```python
from build123d import *

# Parameters (mm, degrees)
CROQUIS1_R              = 37.5
CROQUIS1_R_2            = 35
SALIENTE_EXTRUIR1_DEPTH = 15
CROQUIS2_R              = 40
SALIENTE_EXTRUIR2_DEPTH = 2
CORTAR_EXTRUIR1_DEPTH   = 10
CROQUIS5_W              = 2
CROQUIS5_H              = 4
SALIENTE_EXTRUIR3_START = -2
CROQUIS8_R              = 35
CROQUIS8_R_2            = 34
SALIENTE_EXTRUIR3_DEPTH = 7
REDONDEO1_R             = 0.5


with BuildPart() as part:
    # Croquis1 → Saliente-Extruir1 (new body)
    with BuildSketch(Plane(origin=(0, 17, 0), x_dir=(1, 0, 0), z_dir=(0, 1, 0))):
        with Locations(Location((13.541348433, 6.626768313, 0), (0, 0, 270))):
            Circle(CROQUIS1_R)
        with Locations(Location((13.541348433, 6.626768313, 0), (0, 0, 270))):
            Circle(CROQUIS1_R_2, mode=Mode.SUBTRACT)
    extrude(amount=SALIENTE_EXTRUIR1_DEPTH)

    # Croquis2 → Saliente-Extruir2 (add)
    with BuildSketch(Plane(origin=(0, 32, 0), x_dir=(1, 0, 0), z_dir=(0, 1, 0))):
        with Locations(Location((13.541348433, 6.626768313, 0), (0, 0, 270))):
            Circle(CROQUIS2_R)
    extrude(amount=SALIENTE_EXTRUIR2_DEPTH)

    # Croquis7 → Cortar-Extruir1 (cut)
    with BuildSketch(Plane.XZ.offset(-32)):
        with BuildLine():
            Line((13.541348433, -41.626768313), (13.541348433, -11.626768313))
            ThreePointArc((13.541348433, -11.626768313), (10.005814527, -10.162302219), (8.541348433, -6.626768313))
            Line((8.541348433, -6.626768313), (-21.458651567, -6.626768313))
            ThreePointArc((-21.458651567, -6.626768313), (-11.207388908, -31.375505654), (13.541348433, -41.626768313))
        make_face()
        with BuildLine():
            Line((48.541348433, -6.626768313), (18.541348433, -6.626768313))
            ThreePointArc((18.541348433, -6.626768313), (17.076882339, -3.091234407), (13.541348433, -1.626768313))
            Line((13.541348433, -1.626768313), (13.541348433, 28.373231687))
            ThreePointArc((13.541348433, 28.373231687), (38.290085775, 18.121969029), (48.541348433, -6.626768313))
        make_face()
    extrude(amount=-CORTAR_EXTRUIR1_DEPTH, mode=Mode.SUBTRACT)

    # Cortar-Barrer1: sweep along a path in Croquis6
    with BuildLine(Plane(origin=(0, 33, 0), x_dir=(1, 0, 0), z_dir=(0, 1, 0))) as cortar_barrer1_path:
        CenterArc((13.541348433, 6.626768313), 36.25, 0, 360)
    # Croquis5 → Cortar-Barrer1 (sweep, cut)
    with BuildSketch(Plane.XY.offset(-6.626768313)):
        with Locations((-22.208651567, 32.1)):
            Rectangle(CROQUIS5_W, CROQUIS5_H)
    sweep(path=cortar_barrer1_path.line, mode=Mode.SUBTRACT)


with BuildPart() as cortar_barrer1_piece_1:
    # of the separate pieces the step leaves, piece 1, a body of its own (cortar_barrer1_pieces)
    add(part.part.solids().sort_by_distance((13.541348433, 32, 33.373231687))[0])



with BuildPart() as cortar_barrer1_piece_2:
    # of the separate pieces the step leaves, piece 2, a body of its own (cortar_barrer1_pieces)
    add(part.part.solids().sort_by_distance((18.541348433, 34, -6.626768313))[0])


with BuildPart() as cortar_barrer1_piece_1_1:
    add(cortar_barrer1_piece_1.part)

    add(cortar_barrer1_piece_2.part)  # Saliente-Extruir3 merges Cortar-Barrer1 piece 2
    # Croquis8 → Saliente-Extruir3 (add)
    with BuildSketch(Plane.XZ.offset(-32).offset(SALIENTE_EXTRUIR3_START)):
        with Locations(Location((13.541348433, -6.626768313, 0), (0, 0, 90))):
            Circle(CROQUIS8_R)
        with Locations(Location((13.541348433, -6.626768313, 0), (0, 0, 270))):
            Circle(CROQUIS8_R_2, mode=Mode.SUBTRACT)
    extrude(amount=SALIENTE_EXTRUIR3_DEPTH)

    # Redondeo1
    redondeo1_edges = [cortar_barrer1_piece_1_1.edges().sort_by_distance(p)[0] for p in [
        (13.541348433, 27, 27.373231687),
        (13.541348433, 27, -41.626768313),
    ]]
    fillet(redondeo1_edges, radius=REDONDEO1_R - 0.0001)  # a hair under: the kernel refuses the full size


solid = cortar_barrer1_piece_1_1.part
```
The model under review builds one solid part; all positions refer to its coordinate system, in mm. A direction names the side the tool comes from. Round coordinates to 2 decimals unless told otherwise and drop trailing zeros. Order: outer loops, then holes, each group sorted by start corner. A loop starts at its lowest first (then second) coordinate and runs counter-clockwise, first axis right, second up. Notation, with made-up numbers: M 44.25,2 L 74.25,2 A8 ccw 74.25,13 Z; hole C -23,70.25 d3. An arc over 180 degrees is marked long. Use a Markdown table: item, result.
1) Consider section A-A (y = 22.75). Write out the cut boundary in (x, z), then the cut area to 3 significant figures.
Report:
| item | result |
|---|---|
| outline | C 13.54,-6.63 d75; hole C 13.54,-6.63 d70 |
| area | 569 mm^2 |
2) Insertion check: pin 1 (2 mm diameter, centred on y = 25, z = -17.5, fed in from -X); pin 2 (2 mm diameter, centred on x = 10.5, y = 22, fed in from -Z); pin 3 (1.6 mm diameter, centred on y = 33.5, z = -22, fed in from -X); pin 4 (1.5 mm diameter, centred on x = 11, z = -36, fed in from +Y). Each pin has a flat end and moves straight along its axis. Give the tip position at first contact, or say it passes through.
Report:
| item | result |
|---|---|
| pin 1 | x = -22.64 |
| pin 2 | z = -44.07 |
| pin 3 | x = -23.71 |
| pin 4 | through |
3) Wall thickness on line 1 along X through (y, z) = (31.75, -7.5); line 2 along X through (y, z) = (30.25, -10.5); line 3 along Z through (x, y) = (13, 23.5): over which ranges is each line inside the solid? List them lowest first. Write a range as [from, to].
Report:
| item | result |
|---|---|
| line 1 | [-23.95, -23.2], [-21.45, -20.45], [47.53, 48.53], [50.28, 51.03] |
| line 2 | [-23.76, -23], [-21.24, -20.24], [47.32, 48.33], [50.09, 50.84] |
| line 3 | [-44.12, -41.62], [28.37, 30.87] |
4) Tool access review of faces 1 (the face through (36.52, 30.073, 18.433)), 2 (the face through (33, 33, -6.627)), 3 (the face through (8.757, 32.023, -43.064)): name each direction out of +Z, -Z, +X, -X, +Y, -Y from which nothing blocks a thin tool from reaching the whole face with its end or side.
Report:
| item | result |
|---|---|
| face 1 | -Y |
| face 2 | +Y, -Y |
| face 3 | +Y |
